Geometry: see drawing. Coordinates: mm, zero at the bounding-box minimum. A direction names the side the tool comes from. Round coordinates to 2 decimals unless told otherwise and drop trailing zeros. Order: outer loops, then holes, each group sorted by start corner. A loop starts at its lowest first (then second) coordinate and runs counter-clockwise, first axis right, second up. Notation, with made-up numbers: (52, -31.5) - (65, -31.5) arc R25 cw to (65, 4.5) - close; hole circle Ø2 at (-33.5, 19). An arc over 180 degrees is marked (long way). Put each result on its own line as item: value. Start each with the question number.
1) Section B-B on z = 9.5. Output: boundary loops of the cut face in (x, y).
2) Section C-C on y = 60. Output: boundary loops of the cut face in (x, z), then the cut area to 3 significant figures.
3) Section A-A on x = 47. Output: boundary loops of the cut face in (y, z), then the cut area to 3 significant figures.
4) Mould query, pull axis X, two halves, no side actions, for the marked faces 1, 2, 3 and 4. Classes: +X half, -X half, draft (parallel to the pull), parting line (faces both ways), or undercut.
5) Access query for the marked faces 5, 6 and 7. Directions: +Z, -Z, +X, -X, +Y, -Y. A direction counts if a zero-diameter tool reaches every point of the face in a straight line with its end or side. Return the directions, or none.
6) Line query: probe 1 along Y at (x, z) = (20, 57.5); probe 2 along Y at (x, z) = (90, 23.5); probe 3 along X at (y, z) = (96, 22). Output: solid intervals per line, ascending. Write a range as [from, to].
7) Contact query for flat-ended pins moving along their axis: P1, Ø13, axis at x = 26, y = 30.5, coming from the +Z side; P2, Ø13, axis at x = 23, y = 87.5, coming from the -Z side. Output: stop coordinate, or through.
8) Section D-D on y = 30. Output: boundary loops of the cut face in (x, z).
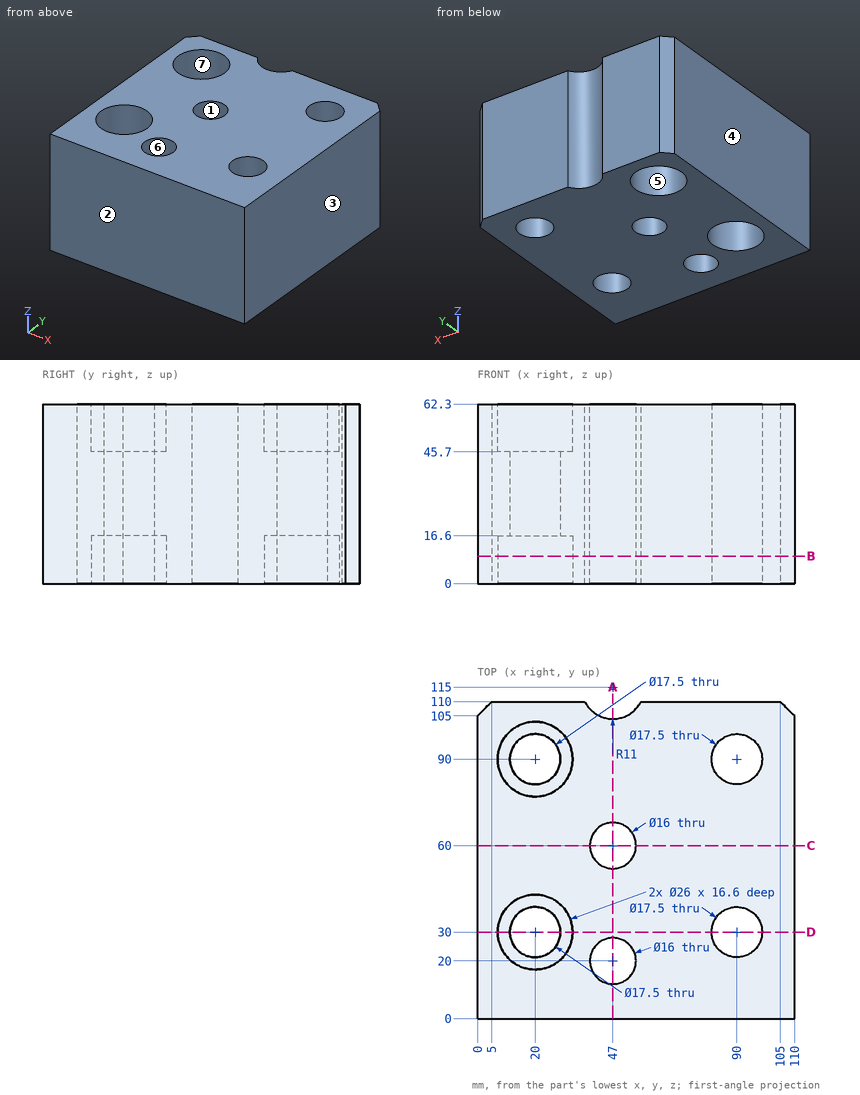
Answer sheet:
1. outline: (0, 0) - (110, 0) - (110, 105) - (105, 110) - (56.8, 110) arc R11 cw to (37.2, 110) - (5, 110) - (0, 105) - close; hole circle Ø26 at (20, 30); hole circle Ø26 at (20, 90); hole circle Ø16 at (47, 20); hole circle Ø16 at (47, 60); hole circle Ø17.5 at (90, 30); hole circle Ø17.5 at (90, 90)
2. outline: (0, 0) - (39, 0) - (39, 62.3) - (0, 62.3) - close; (55, 0) - (110, 0) - (110, 62.3) - (55, 62.3) - close
2. area: 5,860 mm^2
3. outline: (0, 0) - (12, 0) - (12, 62.3) - (0, 62.3) - close; (28, 0) - (52, 0) - (52, 62.3) - (28, 62.3) - close; (68, 0) - (104, 0) - (104, 62.3) - (68, 62.3) - close
3. area: 4,490 mm^2
4. face 1: undercut
4. face 2: draft
4. face 3: +X half
4. face 4: -X half
5. face 5: -Z
5. face 6: +Z, -Z
5. face 7: +Z
6. probe 1: [0, 17], [43, 77], [103, 110]
6. probe 2: [0, 21.25], [38.75, 81.25], [98.75, 110]
6. probe 3: [0, 13.63], [26.37, 83.63], [96.37, 110]
7. P1: z = 45.7
7. P2: z = 16.6
8. outline: (0, 0) - (7, 0) - (7, 16.6) - (11.25, 16.6) - (11.25, 45.7) - (7, 45.7) - (7, 62.3) - (0, 62.3) - close; (28.75, 16.6) - (33, 16.6) - (33, 0) - (81.25, 0) - (81.25, 62.3) - (33, 62.3) - (33, 45.7) - (28.75, 45.7) - close; (98.75, 0) - (110, 0) - (110, 62.3) - (98.75, 62.3) - close
